```python
from build123d import *

# Parameters (mm, degrees)
BOX030_W      = 5
BOX030_H      = 10
BOX030_DEPTH  = 8
BOX029_W      = 5
BOX029_H      = 8
BOX029_DEPTH  = 10
TUBE012_R     = 6
TUBE012_R_2   = 4
TUBE012_DEPTH = 5


with BuildPart() as cube030:
    # Box030 → Box030 (new body)
    with BuildSketch(Plane(origin=(0, -2, 3), x_dir=(1, 0, 0), z_dir=(0, 0, 1))):
        with Locations((2.5, 5)):
            Rectangle(BOX030_W, BOX030_H)
    extrude(amount=BOX030_DEPTH)


with BuildPart() as cube029:
    # Box029 → Box029 (new body)
    with BuildSketch(Plane(origin=(0, 3, -2), x_dir=(1, 0, 0), z_dir=(0, 0, 1))):
        with Locations((2.5, 4)):
            Rectangle(BOX029_W, BOX029_H)
    extrude(amount=BOX029_DEPTH)


with BuildPart() as cut034:
    # Tube012 → Tube012 (new body)
    with BuildSketch(Plane(origin=(0, 3, 3), x_dir=(0, 0, -1), z_dir=(1, 0, 0))):
        Circle(TUBE012_R)
        Circle(TUBE012_R_2, mode=Mode.SUBTRACT)
    extrude(amount=TUBE012_DEPTH)

    # Cut033: cut Cube029
    add(cube029.part, mode=Mode.SUBTRACT)

    # Cut034: cut Cube030
    add(cube030.part, mode=Mode.SUBTRACT)


with BuildPart() as cut034_1:
    # Cut034 placement: moved
    add(cut034.part.moved(Location((0, 1, 1))))


solid = cut034_1.part
```
Verification items for the finished model (mm, model axes). A direction names the side the tool comes from. Give positions to 0.01 mm unless a question says otherwise; leave off trailing zeros. Order: outer loops, then holes, each group sorted by start corner. A loop starts at its lowest first (then second) coordinate and runs counter-clockwise, first axis right, second up. Notation, with made-up numbers: (70, -39.75) - (112, -39.75) arc R10 ccw to (112, -31.75) - close; hole circle Ø11 at (57.5, 8.5). An arc over 180 degrees is marked (long way). Answer as CSV lines item,"result". Start each with the question number.
Item 1: Section check B-B, the plane y = 0.25. Record the boundary of the cut face in (x, z).
Item 2: Section check C-C, the plane z = 1.75. Record the boundary of the cut face in (x, y).
Item 3: Material ranges on L1, parallel to Y at x = 3.3, z = 5; L2, parallel to Z at x = 1.2, y = 4.75; L3, parallel to Z at x = 3.1, y = 3.5, recorded low to high.
Item 4: Gauge pin test, flat ends, axial feed: pin 1 (3 mm diameter, centred on x = 4, y = 3, fed in from +Z); pin 2 (1.7 mm diameter, centred on x = 2.5, y = 5, fed in from +Z); pin 3 (1 mm diameter, centred on x = 2, z = 6, fed in from +Y). Record the tip position at first contact, or that the pin passes through.
Item 5: Access from +Z, -Z, +X, -X, +Y, -Y to the whole of each face (thin tool, end or side, straight path). Record for faces 1 (the face through (2.465, -0.323, -0.16)), 2 (the face through (2.5, -0.5, 4)).
Item 6: Section check A-A, the plane x = 1.45. Record the boundary of the cut face in (y, z).
Filled in:
1,outline,"(0, -0.68) - (5, -0.68) - (5, 2.61) - (0, 2.61) - close"
2,outline,"(0, -1.56) - (5, -1.56) - (5, 0.69) - (0, 0.69) - close"
3,L1,"-1.92 to -1"
3,L2,"-1.95 to -1"
3,L3,"-1.98 to 0.03"
4,pin 1,"z = 0.88"
4,pin 2,"z = -1"
4,pin 3,"y = -1"
5,face 1,"+X, -X"
5,face 2,"+Z, +X, -X, +Y"
6,outline,"(-1, 4) - (-1, 7.32) arc R6 ccw to (7.32, -1) - (4, -1) - (4, 0) arc R4 cw to (0, 4) - close"
